from build123d import *

# Parameters (mm, degrees)
F1_DEPTH       = 30
F2_D           = 6.6
F2_CSINK_D     = 13.44
F2_CSINK_ANGLE = 90


# Not quite as in the source:
# - a feature names something its author has since deleted; it is built from what else it names


with BuildPart() as f1:
    # F0 (on Right) → F1 (new body)
    with BuildSketch(Plane.YZ):
        with BuildLine():
            Line((-278.9958539005, 831.5081800917), (-278.9958539005, -818.4918199083))
            Line((-278.9958539005, -818.4918199083), (321.0041460995, -818.4918199083))
            Line((321.0041460995, -818.4918199083), (321.0041460995, 0))
            Line((321.0041460995, 0), (412.2409460549, 134.0160220861))
            ThreePointArc((412.2409460549, 134.0160220861), (346.0454150195, 328.1386194333), (323.6229111026, 532.0078482247))
            Line((323.6229111026, 532.0078482247), (323.6229111026, 881.5081800917))
            ThreePointArc((323.6229111026, 881.5081800917), (19.1314569656, 894.8597016737), (-278.9958539005, 831.5081800917))
        make_face()
    extrude(amount=F1_DEPTH)

    # F2 (through all)
    with Locations(Plane(origin=(0, 0, 0), x_dir=(0, 1, 0), z_dir=(-1, 0, 0))):
        with Locations((293.6229111026, -742.0078482247), (293.6229111026, -862.0078482247), (229.6229111026, -862.0078482247), (229.6229111026, -742.0078482247), (-248.9958539005, -801.5081800917), (-248.9958539005, -181.5081800917), (306.0041460995, 38.4918199083), (306.0041460995, 348.4918199083), (306.0041460995, 758.4918199083), (306.0041460995, 803.4918199083), (-208.9958539005, 803.4918199083), (-248.9958539005, 788.4918199083), (306.0041460995, 268.4918199083), (318.5190369661, -31.8890116707), (169.7269624564, -133.1852039145), (149.0127494203, -152.9318064879), (70.5869059911, -319.3811593927), (-5.7078003883, -481.3074320555), (-13.9958539005, -520.7695364952), (-13.9958539005, -695.7695364952), (293.033330664, -721.4207649231), (3.033330664, -721.4207649231)):
            CounterSinkHole(F2_D / 2, F2_CSINK_D / 2, counter_sink_angle=F2_CSINK_ANGLE)


solid = f1.part
Can you work these out from the model? Positions are in its coordinate system, mm. A direction names the side the tool comes from. Round coordinates to 2 decimals unless told otherwise and drop trailing zeros. Write each loop counter-clockwise with the first axis right and the second up, starting at its lowest first coordinate (ties: lowest second). Pieces come first, ordered by that corner, then holes. Notation, with made-up numbers: (62.5, -20.75) - (76.5, -20.75) arc R16 ccw to (76.5, 1.25) - close; hole circle Ø3 at (-14, 74). An arc over 180 degrees is marked (long way). Write each question's results on one line, items separated by ' | '. Start each with the question number.
1) Which directions (+Z, -Z, +X, -X, +Y, -Y) give clear straight access to the entire face, cutting with the end or side of a thin tool? Please do faces 1 (the flat face through (15, 17, -818.492)), 2 (the flat face through (15, 321.004, -415)), 3 (the flat face through (15, 323.623, 704)).
2) Suppose I cut it at C-C (y = -156.5). List the corners of the cut face in (x, z) for me, and give its area (3 significant figures).
3) For pin 1 Ø4 at (y, z) = (-14, 695.77) entering from -X; pin 2 Ø7.5 at (y, z) = (-249, -788.49) entering from -X; pin 3 Ø1 at (x, z) = (25, -365.5) entering from +Y, each with a flat end and sliding along its axis, tell me the tip position at first contact or that it passes through.
4) Please list where these lines run through material, in increasing order: line 1 (Z direction, x = 3, y = 232); line 2 (Z direction, x = 24.25, y = -148.5); line 3 (Y direction, x = 2.5, z = 830).
5) Suppose I cut it at A-A (x = 21.75). Give the number of separate pieces and of enclosed holes in the cut face, and give its area (3 significant figures).
6) Suppose I cut it at B-B (z = -641.5). List the corners of the cut face in (x, y) for me, and give its area (3 significant figures).
Here are the results:
1) face 1: -Z, +X, -X, +Y, -Y | face 2: -Z, +X, -X, +Y | face 3: +Z, +X, -X, +Y
2) outline: (0, -818.49) - (30, -818.49) - (30, 867.15) - (0, 867.15) - close | area: 50,600 mm2
3) pin 1: passes through | pin 2: stops at x = 2.97 | pin 3: stops at y = 321
4) line 1: z = -818.49 to 739.15, 744.87 to 859.15, 864.87 to 893.68 | line 2: z = -818.49 to 868.99 | line 3: y = -279 to 323.62
5) separate pieces: 1 | enclosed holes: 22 | area: 1,040,000 mm2
6) outline: (0, -279) - (30, -279) - (30, 321) - (0, 321) - close | area: 18,000 mm2
